Check sheet for the modelled part. Datum: model origin and axes. Units: mm. Face numbers are marked on the shaded views. Give positions to 0.01 mm unless a question says otherwise; leave off trailing zeros. Order: outer loops, then holes, each group sorted by start corner. A loop starts at its lowest first (then second) coordinate and runs counter-clockwise, first axis right, second up.
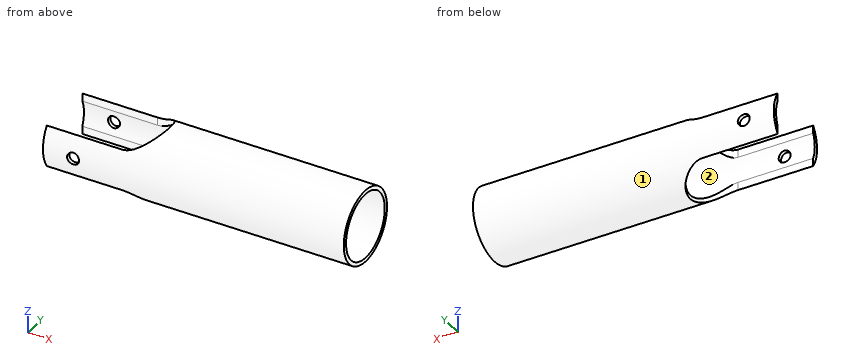
from build123d import *

# Parameters (mm, degrees)
SKETCH1_R               = 1.2065
SKETCH1_R_2             = 1.0795
BOSS_EXTRUDE1_DEPTH     = 10
CUT_EXTRUDE1_DEPTH      = 10
CUT_EXTRUDE1_DEPTH_BACK = 1.5
SKETCH4_R               = 0.1984375
CUT_EXTRUDE2_DEPTH      = 5
CUT_EXTRUDE2_DEPTH_BACK = 5


with BuildPart() as part:
    # Sketch1 → Boss-Extrude1 (new body)
    with BuildSketch(Plane(origin=(0, 0, 0), x_dir=(0, 0, -1), z_dir=(1, 0, 0))):
        Circle(SKETCH1_R)
        Circle(SKETCH1_R_2, mode=Mode.SUBTRACT)
    extrude(amount=BOSS_EXTRUDE1_DEPTH)

    # Sketch2 → Cut-Extrude1 (cut, two sides)
    with BuildSketch(Plane.XY) as cut_extrude1_sk:
        with BuildLine():
            Line((2.5, -0.9921875), (0, -0.9921875))
            Line((0, -0.9921875), (0, 0.9921875))
            Line((0, 0.9921875), (2.5, 0.9921875))
            ThreePointArc((2.5, 0.9921875), (3.4921875, 0), (2.5, -0.9921875))
        make_face()
    extrude(amount=CUT_EXTRUDE1_DEPTH, mode=Mode.SUBTRACT)
    extrude(cut_extrude1_sk.sketch, amount=-CUT_EXTRUDE1_DEPTH_BACK, mode=Mode.SUBTRACT)

    # Sketch4 → Cut-Extrude2 (cut, two sides)
    with BuildSketch(Plane(origin=(0, 0, 0), x_dir=(1, 0, 0), z_dir=(0, 1, 0))) as cut_extrude2_sk:
        with Locations((1, 0)):
            Circle(SKETCH4_R)
    extrude(amount=CUT_EXTRUDE2_DEPTH, mode=Mode.SUBTRACT)
    extrude(cut_extrude2_sk.sketch, amount=-CUT_EXTRUDE2_DEPTH_BACK, mode=Mode.SUBTRACT)


solid = part.part
1) Section check B-B, the plane z = 0. Record the cut outline in (x, y).
Recorded:
outline: (0, -1.21) - (0.8, -1.21) - (0.8, -1.08) - (0, -1.08) - close; (0, 1.08) - (0.8, 1.08) - (0.8, 1.21) - (0, 1.21) - close; (1.2, -1.21) - (10, -1.21) - (10, -1.08) - (1.2, -1.08) - close; (1.2, 1.08) - (10, 1.08) - (10, 1.21) - (1.2, 1.21) - close
2) Draft check along Y on the marked faces 1 and 2. Enter one of: +Y half, -Y half, draft (parallel to the pull), parting line (faces both ways), or undercut.
Recorded:
face 1: parting line
face 2: undercut
3) Section check C-C, the plane x = 2. Record the cut outline in (y, z).
Recorded:
outline: (-0.99, -0.69) - (-0.99, -0.43) arc R1.08 cw to (-0.99, 0.43) - (-0.99, 0.69) arc R1.21 ccw to start; (0.99, -0.69) arc R1.21 ccw to (0.99, 0.69) - (0.99, 0.43) arc R1.08 cw to (0.99, -0.43) - close
4) Section check D-D, the plane z = 0.55. Record the cut outline in (x, y).
Recorded:
outline: (0, -1.07) - (10, -1.07) - (10, -0.93) - (2.85, -0.93) arc R0.99 cw to (2.5, -0.99) - (0, -0.99) - close; (0, 0.99) - (2.5, 0.99) arc R0.99 cw to (2.85, 0.93) - (10, 0.93) - (10, 1.07) - (0, 1.07) - close
5) Material ranges on L1, parallel to X at y = -1.15, z = 0; L2, parallel to Y at x = 5.5, z = -0.65; L3, parallel to Z at x = 1, y = 1.1, recorded low to high.
Recorded:
L1: x = 0 to 0.8, 1.2 to 10
L2: y = -1.02 to -0.86, 0.86 to 1.02
L3: z = -0.5 to -0.2, 0.2 to 0.5
6) Section check A-A, the plane y = 0. Record the cut outline in (x, z), then the cut area to 3 significant figures.
Recorded:
outline: (3.49, -1.21) - (10, -1.21) - (10, -1.08) - (3.49, -1.08) - close; (3.49, 1.08) - (10, 1.08) - (10, 1.21) - (3.49, 1.21) - close
area: 1.65 mm2
